For this review, take the finished solid that the model builds, in its own axes (mm). Give positions to 0.01 mm unless a question says otherwise; leave off trailing zeros. Loops run counter-clockwise (first coordinate to the right, second up) from the corner with the lowest first, then second, coordinate; pieces in that order, holes last.
```python
from build123d import *

# Parameters (mm, degrees)
F0_W     = 38.1
F0_H     = 42.037
F1_DEPTH = 15.875
F3_D     = 4


with BuildPart() as f1:
    # F0 (on Front) → F1 (new body)
    with BuildSketch(Plane.XZ):
        with Locations((-7.488622, 21.0185)):
            Rectangle(F0_W, F0_H)
    extrude(amount=F1_DEPTH)

    # F3 (through all)
    with Locations(Plane(origin=(0, 0, 0), x_dir=(1, 0, 0), z_dir=(0, 0, -1))):
        with Locations((-7.88276, 7.485884), (-21.808967, 6.43485)):
            Hole(F3_D / 2)


solid = f1.part
```
Item 1: Clearance check with flat-ended pins moving along their axes: pin 1 Ø1 at (x, y) = (-4.5, -10.5) entering from -Z; pin 2 Ø3.5 at (x, y) = (-7.88, -7.49) entering from -Z. State where each tip first meets the part, or that it passes through.
Answer:
pin 1: stops at z = 0
pin 2: passes through
Item 2: Take a section at A-A on z = 16. Give the boundary of the cut face in (x, y) (3 decimals), and give its area (3 significant figures).
Answer:
outline: (-26.539, -15.875) - (11.561, -15.875) - (11.561, 0) - (-26.539, 0) - close; hole circle Ø4 at (-21.809, -6.435); hole circle Ø4 at (-7.883, -7.486)
area: 580 mm2
Item 3: The part is to be moulded in two halves that separate along X. For faces 1 (the flat face through (11.561, -8, 21)), 2 (the flat face through (-8, -10, 0)), 3 (the cylindrical face through (-9.79, -8.09, 21.31)), say which applies: released by +X, released by -X, zero draft, split by the parting line, or undercut.
Answer:
face 1: released by +X
face 2: zero draft
face 3: undercut
Item 4: For L1, parallel to X at y = -6.25, z = 32; L2, parallel to Y at x = -22, z = 19.5 (3 decimals); L3, parallel to Y at x = -8.5, z = 23.5 (3 decimals), list the stretches that pass through material, from the lowest coordinate up.
Answer:
L1: x = -26.54 to -23.8, -19.82 to -9.46, -6.31 to 11.56
L2: y = -15.875 to -8.426, -4.444 to 0
L3: y = -15.875 to -9.388, -5.584 to 0
